Autodesk Inventor part; units mm, degrees
ref_plane "YZ Plane" through (0, 0, 0) normal (1, 0, 0) x (0, 1, 0)
ref_plane "XZ Plane" through (0, 0, 0) normal (0, 1, 0) x (-1, 0, 0)
ref_plane "XY Plane" through (0, 0, 0) normal (0, 0, 1) x (1, 0, 0)
sketch "Sketch1" plane through (0, 0, 0) normal (0, 1, 0) x (-1, 0, 0)
  line L0 (0, 0) -> (40, 0)
  line L1 (40, 0) -> (40, -9.797)
  line L2 (40, -9.797) -> (0, -9.797)
  line L3 (0, -9.797) -> (0, 0)
  circle A0 centre (7.813, -4.8985) radius 3
  dimension "d1" = 40
  dimension "d3" = 6
extrude "Extrusion1" add sketch "Sketch1" along normal blind 6
equation "\"BendRadius\" = Thickness"
equation "\"BendReliefWidth\" = Thickness"
equation "\"BendReliefDepth\" = 0.5 * Thickness"
equation "\"CornerReliefSize\" = 4 * Thickness"
equation "\"MinimumRemnant\" = 2 * Thickness"
equation "\"TransitionRadius\" = BendRadius"
equation "\"JacobiRadiusSize\" = BendRadius"
equation "\"GapSize\" = Thickness"
Read the model definition and answer for the solid it produces. Units are mm, in the model's axes. Give positions to 0.01 mm unless a question says otherwise; leave off trailing zeros. Write each loop counter-clockwise with the first axis right and the second up, starting at its lowest first coordinate (ties: lowest second). Pieces come first, ordered by that corner, then holes. Notation, with made-up numbers: (73, 56.25) - (130, 56.25) arc R25 ccw to (130, 69.25) - close; hole circle Ø6 at (43.25, 43). An arc over 180 degrees is marked (long way). Return JSON: item names as keys, results as strings.
Q1. A cutting plane is placed at A-A, the plane z = -6. Determine the outline of the cut face in (x, y).
Reply:
{"outline": "(-40, 0) - (-10.6, 0) - (-10.6, 6) - (-40, 6) - close; (-5.02, 0) - (0, 0) - (0, 6) - (-5.02, 6) - close"}
Q2. A cutting plane is placed at C-C, the plane y = 2.7. Determine the outline of the cut face in (x, z).
Reply:
{"outline": "(-40, -9.8) - (0, -9.8) - (0, 0) - (-40, 0) - close; hole circle Ø6 at (-7.81, -4.9)"}
Q3. Given P1, Ø3, axis at x = -7.5, z = -4, coming from the +Y side, flat-ended and moving along its own axis, determine where the tip first touches the part or whether it passes through.
Reply:
{"P1": "through"}
Q4. For a pull along Z with two mould halves and no side action, classify faces 1 (the face through (-20, 3, -9.797)), 2 (the face through (-9.2, 2.96, -2.24)), 3 (the face through (-20, 0, -5)), 4 (the face through (-20, 3, 0)) as released by +Z, released by -Z, zero draft, split by the parting line, or undercut.
Reply:
{"face 1": "released by -Z", "face 2": "undercut", "face 3": "zero draft", "face 4": "released by +Z"}
Q5. Consider line 1 along Z through (x, y) = (-8, 2.3); line 2 along X through (y, z) = (1.35, -4.75); line 3 along X through (y, z) = (3.5, -3.75). Determine where each line is inside the solid, lowest interval first. Write a range as [from, to].
Reply:
{"line 1": "[-9.8, -7.89], [-1.9, 0]", "line 2": "[-40, -10.81], [-4.82, 0]", "line 3": "[-40, -10.58], [-5.04, 0]"}
Q6. A cutting plane is placed at B-B, the plane x = -9.5. Determine the outline of the cut face in (y, z), and give its area (3 significant figures).
Reply:
{"outline": "(0, -9.8) - (6, -9.8) - (6, -7.38) - (0, -7.38) - close; (0, -2.42) - (6, -2.42) - (6, 0) - (0, 0) - close", "area": "29.0 mm²"}
